Part model, mm, in its own coordinate system. A direction names the side the tool comes from. Coordinates: 2 decimals unless noted, no trailing zeros. Order: outer loops, then holes, each group sorted by start corner. A loop starts at its lowest first (then second) coordinate and runs counter-clockwise, first axis right, second up. Notation, with made-up numbers: (-16.75, -28) - (28.25, -28) arc R17 cw to (28.25, -23) - close; hole circle Ø7 at (10.5, 40.25). An arc over 180 degrees is marked (long way). Use a Markdown table: item, result. Add a question column.
1) Saw through at C-C on y = -19.5. List the corners of the cut face in (x, z).
2) Two-plate mould, pull along Z, no slides. Class faces 6 (the face through (0, -12, 1)), 7 (the face through (6, -12, -6.1)), 8 (the face through (15, -12, -4)): +Z half, -Z half, draft (parallel to the pull), parting line (faces both ways), or undercut.
3) Wall check: L1, parallel to Y at x = 5.5, z = -4.8; L2, parallel to Z at x = 7.5, y = -4; L3, parallel to Z at x = 10, y = -21.75. Give the ranges that are in metal, low to high. Write a range as [from, to].
4) Saw through at B-B on z = -4.25. List the corners of the cut face in (x, y), then the cut area to 3 significant figures.
5) Saw through at A-A on x = 2.5. List the corners of the cut face in (y, z), then the cut area to 4 significant figures.
6) Tool access for faces 1 (the face through (6.6, -24.5, -5.6)), 2 (the face through (5, -14.5, 5)), 3 (the face through (-2, -24.5, 0.1)), 4 (the face through (10, -7, 5)), 5 (the face through (8, -12, -3.6)): list every direction of +Z, -Z, +X, -X, +Y, -Y with a clear straight run to the whole face (end or side of a thin tool).
7) Drop flat-ended pins along their axis: P1, Ø1, axis at y = -20.5, z = 2.5, coming from the +X side; P2, Ø1.8, axis at x = 5.5, y = -19.5, coming from the +Z side; P3, Ø0.7, axis at x = 3.5, z = 4.5, coming from the -Y side; P4, Ø6, axis at y = -11.5, z = 4.5, coming from the +X side. Give the stop position or say it passes through.
8) Saw through at D-D on x = 5.5. List the corners of the cut face in (y, z).
```python
from build123d import *

# Parameters (mm, degrees)
F1_DEPTH = 25
F2_R     = 1.5
F3_DEPTH = 25
F4_W     = 10
F4_H     = 10.5
F4_R     = 1.5
F5_DEPTH = 5
F6_SIZE  = 1


with BuildPart() as f1:
    # F0 (on Front) → F1 (new body)
    with BuildSketch(Plane.XZ):
        Polygon((0, -3.6), (0, 3.6), (10, 3.6), (10, 6.1), (-2.5, 6.1), (-2.5, -6.1), (15, -6.1), (15, -3.6), align=None)
    extrude(amount=F1_DEPTH)

    # F2 (on face) → F3 (cut)
    with BuildSketch(Plane.XY.offset(6.1)):
        with Locations((5.5, -19.5)):
            Circle(F2_R)
    extrude(amount=-F3_DEPTH, mode=Mode.SUBTRACT)

    # F4 (on face) → F5 (cut)
    with BuildSketch(Plane.XY.offset(6.1)):
        with Locations((5, -19.75)):
            Rectangle(F4_W, F4_H)
        with Locations((5.5, -19.5)):
            Circle(F4_R, mode=Mode.SUBTRACT)
    extrude(amount=-F5_DEPTH, mode=Mode.SUBTRACT)

    # F6
    f6_edges = [f1.edges().sort_by_distance(p)[0] for p in [
        (15, -12.5, -6.1),
        (6.25, 0, -6.1),
        (6.25, -25, -6.1),
        (-2.5, -12.5, 6.1),
        (-1.25, -25, 6.1),
        (-2.5, -25, 0),
        (-2.5, 0, 0),
        (-2.5, -12.5, -6.1),
    ]]
    chamfer(f6_edges, length=F6_SIZE)


solid = f1.part
```
Results are:
| question | item | result |
|---|---|---|
| 1 | outline | (-2.5, -5.1) - (-1.5, -6.1) - (4, -6.1) - (4, -3.6) - (0, -3.6) - (0, 6.1) - (-1.5, 6.1) - (-2.5, 5.1) - close; (7, -6.1) - (14, -6.1) - (15, -5.1) - (15, -3.6) - (7, -3.6) - close |
| 2 | face 6 | undercut |
| 2 | face 7 | -Z half |
| 2 | face 8 | draft |
| 3 | L1 | [-25, -21], [-18, 0] |
| 3 | L2 | [-6.1, -3.6], [3.6, 6.1] |
| 3 | L3 | [-6.1, -3.6] |
| 4 | outline | (-2.5, -24) - (-1.5, -25) - (15, -25) - (15, 0) - (-1.5, 0) - (-2.5, -1) - close; hole circle Ø3 at (5.5, -19.5) |
| 4 | area | 429 mm2 |
| 5 | outline | (-25, -5.1) - (-24, -6.1) - (-1, -6.1) - (0, -5.1) - (0, -3.6) - (-25, -3.6) - close; (-14.5, 3.6) - (0, 3.6) - (0, 6.1) - (-14.5, 6.1) - close |
| 5 | area | 97.75 mm2 |
| 6 | face 1 | -Z, +X, -X, -Y |
| 6 | face 2 | +Z, +X, -Y |
| 6 | face 3 | +Z, -Z, -X, -Y |
| 6 | face 4 | +Z, +X, +Y, -Y |
| 6 | face 5 | +X, +Y, -Y |
| 7 | P1 | x = 0 |
| 7 | P2 | through |
| 7 | P3 | y = -14.5 |
| 7 | P4 | x = 10 |
| 8 | outline | (-25, -5.1) - (-24, -6.1) - (-21, -6.1) - (-21, -3.6) - (-25, -3.6) - close; (-18, -6.1) - (-1, -6.1) - (0, -5.1) - (0, -3.6) - (-18, -3.6) - close; (-14.5, 3.6) - (0, 3.6) - (0, 6.1) - (-14.5, 6.1) - close |
